from build123d import *

# Parameters (mm, degrees)
F0_W     = 105
F0_H     = 70
F1_DEPTH = 50
F2_T     = -2.5
F3_R     = 67.5
F3_W     = 105
F3_H     = 70
F4_DEPTH = 5
F5_R     = 2.5
F6_DEPTH = 102.501


with BuildPart() as f1:
    # F0 (on Top) → F1 (new body)
    with BuildSketch(Plane.XY):
        Rectangle(F0_W, F0_H)
    extrude(amount=F1_DEPTH)

    # F2
    f2_openings = [f1.faces().sort_by_distance(p)[0] for p in [
        (0, 0, 50),
    ]]
    offset(amount=F2_T, openings=f2_openings)

    # F3 (on face) → F4 (join)
    with BuildSketch(Plane.XY.offset(50)):
        Circle(F3_R)
        Rectangle(F3_W, F3_H, mode=Mode.SUBTRACT)
    extrude(amount=-F4_DEPTH)

    # F5 (on face) → F6 (cut, through all)
    with BuildSketch(Plane.XZ.offset(35)):
        with Locations((0, 22)):
            Circle(F5_R)
    extrude(amount=-F6_DEPTH, mode=Mode.SUBTRACT)


solid = f1.part
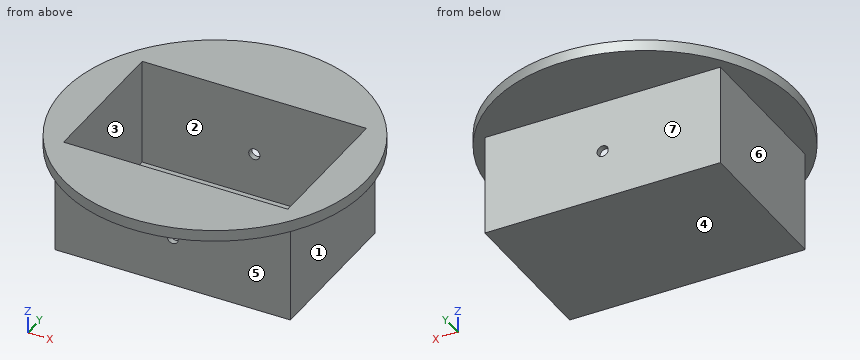
Work out the finished part from the listing and answer in its coordinate system (mm). Face numbers are marked on the shaded views. A direction names the side the tool comes from. Coordinates: 2 decimals unless noted, no trailing zeros. Order: outer loops, then holes, each group sorted by start corner. A loop starts at its lowest first (then second) coordinate and runs counter-clockwise, first axis right, second up. Notation, with made-up numbers: (18.5, -11) - (27.5, -11) arc R37 ccw to (27.5, 25) - close; hole circle Ø4 at (44, -25.75). An arc over 180 degrees is marked (long way). Put each result on its own line as item: value. Start each with the question number.
1) Flat-ended cylindrical pins translate along their axes: pin 1 (22.5 mm diameter, centred on y = -3, z = 24.5, fed in from -X); pin 2 (10 mm diameter, centred on x = -33, y = -46.5, fed in from -Z); pin 3 (3 mm diameter, centred on x = 0, z = 22, fed in from +Y); pin 4 (1 mm diameter, centred on x = -16.5, y = -12.5, fed in from +Z). Find the tip coordinate at first contact, or state that the pin passes through.
2) Find the intervals of material crossed by line 1 (Z direction, x = 0, y = 34.3); line 2 (Y direction, x = 33, z = 8.5); line 3 (X direction, y = 25.5, z = 7.5), in increasing order. Write a range as from..to.
3) Find section A-A (x = 0). Give the vertices of the cut face in (y, z), plus the area to 4 significant figures.
4) Find section B-B (z = 22). Give the vertices of the cut face in (x, y).
5) Find section C-C (y = 0). Give the vertices of the cut face in (x, z).
6) For the marked faces 5, 6 and 7, determine the directions among +Z, -Z, +X, -X, +Y, -Y from which every point of the face is accessible in a straight line to the end or side of a thin tool.
7) Find section D-D (z = 30.5). Give the vertices of the cut face in (x, y), plus the area to 3 significant figures.
8) For a pull along X with two mould halves and no side action, classify the marked faces 1, 2, 3 and 4 as released by +X, released by -X, zero draft, split by the parting line, or undercut.
Results list:
1. pin 1: stops at x = -52.5
1. pin 2: stops at z = 45
1. pin 3: passes through
1. pin 4: stops at z = 2.5
2. line 1: z = 0..19.5, 24.5..50
2. line 2: y = -35..-32.5, 32.5..35
2. line 3: x = -52.5..-50, 50..52.5
3. outline: (-67.5, 45) - (-35, 45) - (-35, 24.5) - (-32.5, 24.5) - (-32.5, 50) - (-67.5, 50) - close; (-35, 0) - (35, 0) - (35, 19.5) - (32.5, 19.5) - (32.5, 2.5) - (-32.5, 2.5) - (-32.5, 19.5) - (-35, 19.5) - close; (32.5, 24.5) - (35, 24.5) - (35, 45) - (67.5, 45) - (67.5, 50) - (32.5, 50) - close
3. area: 712.5 mm^2
4. outline: (-52.5, -35) - (-2.5, -35) - (-2.5, -32.5) - (-50, -32.5) - (-50, 32.5) - (-2.5, 32.5) - (-2.5, 35) - (-52.5, 35) - close; (2.5, -35) - (52.5, -35) - (52.5, 35) - (2.5, 35) - (2.5, 32.5) - (50, 32.5) - (50, -32.5) - (2.5, -32.5) - close
5. outline: (-67.5, 45) - (-52.5, 45) - (-52.5, 0) - (52.5, 0) - (52.5, 45) - (67.5, 45) - (67.5, 50) - (50, 50) - (50, 2.5) - (-50, 2.5) - (-50, 50) - (-67.5, 50) - close
6. face 5: -Z, +X, -X, -Y
6. face 6: -Z, -X, +Y, -Y
6. face 7: -Z, +X, -X, +Y
7. outline: (-52.5, -35) - (52.5, -35) - (52.5, 35) - (-52.5, 35) - close; hole (-50, -32.5) - (50, -32.5) - (50, 32.5) - (-50, 32.5) - close
7. area: 850 mm^2
8. face 1: released by +X
8. face 2: undercut
8. face 3: undercut
8. face 4: zero draft
